Here's how the part is built. I have some questions about the finished solid (model axes, mm). Round coordinates to 2 decimals unless told otherwise and drop trailing zeros. Order: outer loops, then holes, each group sorted by start corner. A loop starts at its lowest first (then second) coordinate and runs counter-clockwise, first axis right, second up. Notation, with made-up numbers: (55, -35) -> (72, -35) arc R24 ccw to (72, -17) -> close; hole circle Ø8 at (51.25, -32). An arc over 180 degrees is marked (long way). Answer in a Markdown table with one row per item.
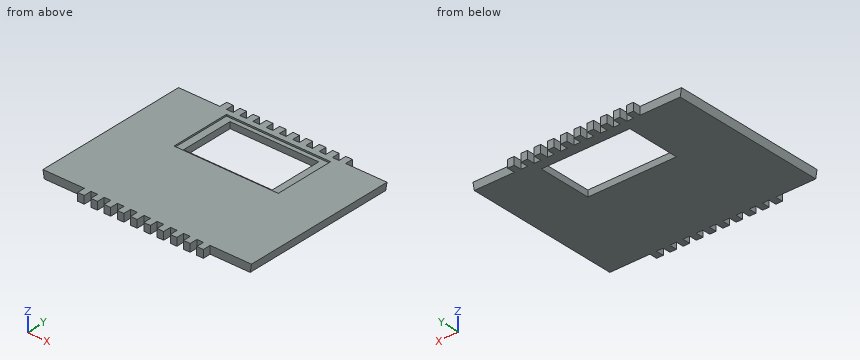
```python
from build123d import *

# Parameters (mm, degrees)
F0_W     = 12.7
F0_H     = 15
F1_DEPTH = 15
F3_DEPTH = 315.001
F5_DEPTH = 315.001
F6_W     = 170
F6_H     = 103
F7_DEPTH = 15
F8_W     = 200
F8_H     = 116
F8_W_2   = 170
F8_H_2   = 103
F9_DEPTH = 3


with BuildPart() as f1:
    # F0 (on Top) → F1 (new body)
    with BuildSketch(Plane.XY):
        Polygon((120.65, -150), (200, -150), (200, 150), (120.65, 150), (107.95, 150), (95.25, 150), (82.55, 150), (69.85, 150), (57.15, 150), (44.45, 150), (31.75, 150), (19.05, 150), (6.35, 150), (0, 150), (-6.35, 150), (-19.05, 150), (-31.75, 150), (-44.45, 150), (-57.15, 150), (-69.85, 150), (-82.55, 150), (-95.25, 150), (-107.95, 150), (-120.65, 150), (-200, 150), (-200, -150), (-120.65, -150), (-107.95, -150), (-95.25, -150), (-82.55, -150), (-69.85, -150), (-57.15, -150), (-44.45, -150), (-31.75, -150), (-19.05, -150), (-6.35, -150), (0, -150), (6.35, -150), (19.05, -150), (31.75, -150), (44.45, -150), (57.15, -150), (69.85, -150), (82.55, -150), (95.25, -150), (107.95, -150), align=None)
        with Locations((-38.1, -157.5)):
            Rectangle(F0_W, F0_H)
        with Locations((114.3, 157.5)):
            Rectangle(F0_W, F0_H)
        with Locations((-114.3, -157.5)):
            Rectangle(F0_W, F0_H)
        with Locations((114.3, -157.5)):
            Rectangle(F0_W, F0_H)
        with Locations((12.7, -157.5)):
            Rectangle(F0_W, F0_H)
        with Locations((63.5, -157.5)):
            Rectangle(F0_W, F0_H)
        with Locations((-63.5, -157.5)):
            Rectangle(F0_W, F0_H)
        with Locations((-63.5, 157.5)):
            Rectangle(F0_W, F0_H)
        with Locations((12.7, 157.5)):
            Rectangle(F0_W, F0_H)
        with Locations((-88.9, 157.5)):
            Rectangle(F0_W, F0_H)
        with Locations((-88.9, -157.5)):
            Rectangle(F0_W, F0_H)
        with Locations((38.1, 157.5)):
            Rectangle(F0_W, F0_H)
        with Locations((88.9, -157.5)):
            Rectangle(F0_W, F0_H)
        with Locations((38.1, -157.5)):
            Rectangle(F0_W, F0_H)
        with Locations((-38.1, 157.5)):
            Rectangle(F0_W, F0_H)
        with Locations((-114.3, 157.5)):
            Rectangle(F0_W, F0_H)
        with Locations((88.9, 157.5)):
            Rectangle(F0_W, F0_H)
        with Locations((63.5, 157.5)):
            Rectangle(F0_W, F0_H)
        with Locations((-12.7, 157.5)):
            Rectangle(F0_W, F0_H)
        with Locations((-12.7, -157.5)):
            Rectangle(F0_W, F0_H)
    extrude(amount=F1_DEPTH)

    # F2 (on face) → F3 (cut, through all)
    with BuildSketch(Plane.XZ.offset(150)):
        Polygon((-200, 0), (-197.500259, 0), (-200, 15), align=None)
    extrude(amount=-F3_DEPTH, mode=Mode.SUBTRACT)

    # F4 (on face) → F5 (cut, through all)
    with BuildSketch(Plane.XZ.offset(150)):
        Polygon((200, 15), (197.505116, 0), (200, 0), align=None)
    extrude(amount=-F5_DEPTH, mode=Mode.SUBTRACT)

    # F6 (on face) → F7 (cut)
    with BuildSketch(Plane.XY.offset(15)):
        with Locations((0, 80)):
            Rectangle(F6_W, F6_H)
    extrude(amount=-F7_DEPTH, mode=Mode.SUBTRACT)

    # F8 (on face) → F9 (cut)
    with BuildSketch(Plane.XY.offset(15)):
        with Locations((1, 81.5)):
            Rectangle(F8_W, F8_H)
        with Locations((0, 80)):
            Rectangle(F8_W_2, F8_H_2, mode=Mode.SUBTRACT)
    extrude(amount=-F9_DEPTH, mode=Mode.SUBTRACT)


solid = f1.part
```
1. Please list where these lines run through material, in increasing order: line 1 along Y through (x, z) = (32.5, 7.5); line 2 along Y through (x, z) = (79.5, 3); line 3 along Y through (x, z) = (-97, 5.25).
Numbers:
| item | result |
|---|---|
| line 1 | y = -165 to 28.5, 131.5 to 165 |
| line 2 | y = -150 to 28.5, 131.5 to 150 |
| line 3 | y = -150 to 150 |
2. Suppose I cut it at B-B on x = -2. Write out the boundary of the cut face in (y, z), then the cut area to 3 significant figures.
Numbers:
| item | result |
|---|---|
| outline | (-150, 0) -> (28.5, 0) -> (28.5, 12) -> (23.5, 12) -> (23.5, 15) -> (-150, 15) -> close; (131.5, 0) -> (150, 0) -> (150, 15) -> (139.5, 15) -> (139.5, 12) -> (131.5, 12) -> close |
| area | 2,920 mm2 |
3. Suppose I cut it at A-A on y = 48.5. Write out the boundary of the cut face in (x, z).
Numbers:
| item | result |
|---|---|
| outline | (-200, 15) -> (-197.5, 0) -> (-85, 0) -> (-85, 12) -> (-99, 12) -> (-99, 15) -> close; (85, 0) -> (197.51, 0) -> (200, 15) -> (101, 15) -> (101, 12) -> (85, 12) -> close |
4. For pin 1 Ø4.5 at (y, z) = (156.5, 6) entering from -X; pin 2 Ø4.5 at (y, z) = (-161, 5.5) entering from +X; pin 3 Ø2 at (y, z) = (119.5, 12.5) entering from +X, each with a flat end and sliding along its axis, tell me the tip position at first contact or that it passes through.
Numbers:
| item | result |
|---|---|
| pin 1 | stops at x = -120.65 |
| pin 2 | stops at x = 120.65 |
| pin 3 | stops at x = 199.75 |
5. Suppose I cut it at C-C on x = -174. Write out the boundary of the cut face in (y, z).
Numbers:
| item | result |
|---|---|
| outline | (-150, 0) -> (150, 0) -> (150, 15) -> (-150, 15) -> close |
